Could you check a few things on this drawing? It's one solid part, dimensions in mm from its lowest x, y, z. A direction names the side the tool comes from. Coordinates: 2 decimals unless noted, no trailing zeros. Order: outer loops, then holes, each group sorted by start corner. A loop starts at its lowest first (then second) coordinate and runs counter-clockwise, first axis right, second up. Notation, with made-up numbers: (23, 73.5) -> (39, 73.5) arc R32 cw to (39, 105.5) -> close; hole circle Ø2 at (-30.5, 10.25). An arc over 180 degrees is marked (long way). Answer as CSV lines item,"result".
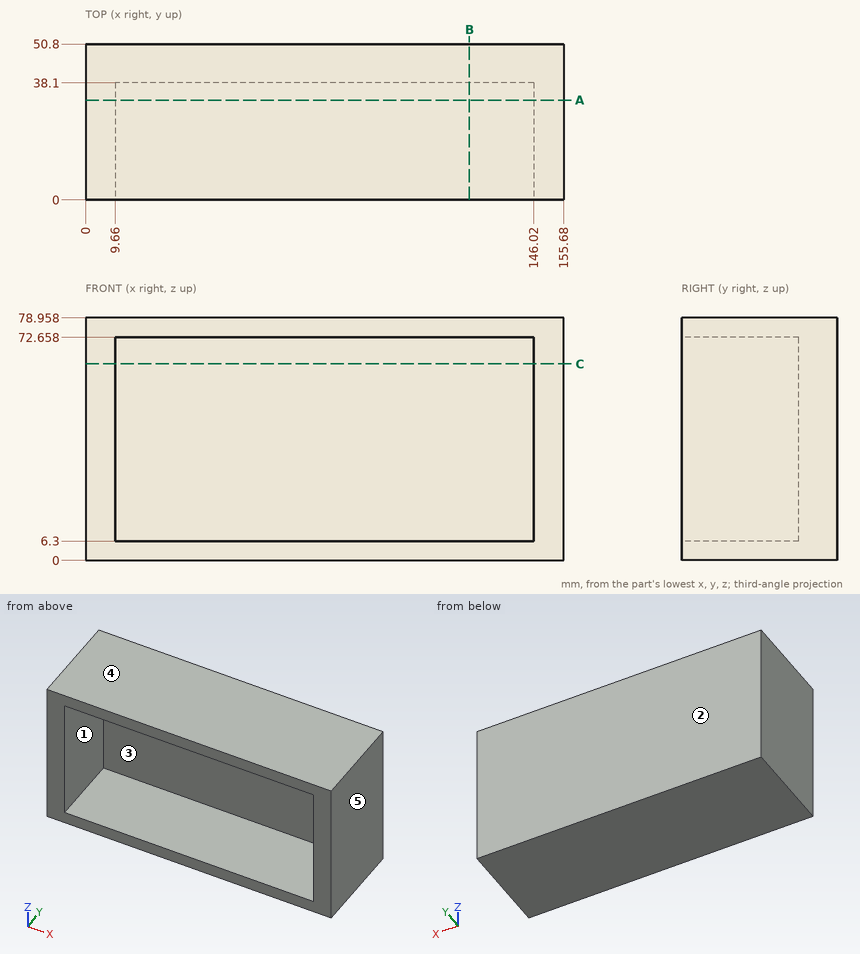
Q1. We'd pull the mould along X, two halves only. Please class the marked faces 3, 4 and 5: pulls with the +X half, pulls with the -X half, needs draft (parallel to the pull), parting line crosses it, or undercut.
Solution:
face 3,"undercut"
face 4,"needs draft"
face 5,"pulls with the +X half"
Q2. For P1, Ø6, axis at x = 70, z = 31.5, coming from the -Y side, with a flat end and sliding along its axis, tell me the tip position at first contact or that it passes through.
Solution:
P1,"y = 38.1"
Q3. Which directions (+Z, -Z, +X, -X, +Y, -Y) give clear straight access to the entire face, cutting with the end or side of a thin tool? Please do the marked faces 1 and 2.
Solution:
face 1,"-Y"
face 2,"+Z, -Z, +X, -X, +Y"
Q4. Imagine slicing it at C-C (z = 64). List the corners of the cut face in (x, y) for me, and give its area (3 significant figures).
Solution:
outline,"(0, 0) -> (9.66, 0) -> (9.66, 38.1) -> (146.02, 38.1) -> (146.02, 0) -> (155.68, 0) -> (155.68, 50.8) -> (0, 50.8) -> close"
area,"2,710 mm2"
Q5. If I drill on line 1 (Z direction, x = 63, y = 2); line 2 (X direction, y = 20.5, z = 47.5); line 3 (Y direction, x = 63.5, z = 36), over which ranges is the centre line in solid material (lowest first)?
Solution:
line 1,"0 to 6.3, 72.66 to 78.96"
line 2,"0 to 9.66, 146.02 to 155.68"
line 3,"38.1 to 50.8"
Q6. Imagine slicing it at B-B (x = 125). List the corners of the cut face in (y, z) for me, and give its area (3 significant figures).
Solution:
outline,"(0, 0) -> (50.8, 0) -> (50.8, 78.96) -> (0, 78.96) -> (0, 72.66) -> (38.1, 72.66) -> (38.1, 6.3) -> (0, 6.3) -> close"
area,"1,480 mm2"
Q7. Imagine slicing it at A-A (y = 32.5). List the corners of the cut face in (x, z) for me.
Solution:
outline,"(0, 0) -> (155.68, 0) -> (155.68, 78.96) -> (0, 78.96) -> close; hole (9.66, 6.3) -> (146.02, 6.3) -> (146.02, 72.66) -> (9.66, 72.66) -> close"
